Here's how the part is built. I have some questions about the finished solid (model axes, mm). A direction names the side the tool comes from. Round coordinates to 2 decimals unless told otherwise and drop trailing zeros. Write each loop counter-clockwise with the first axis right and the second up, starting at its lowest first coordinate (ties: lowest second). Pieces come first, ordered by that corner, then holes. Notation, with made-up numbers: (9.25, 48) - (31.25, 48) arc R30 cw to (31.25, 71) - close; hole circle Ø8 at (76.25, 38.5). An arc over 180 degrees is marked (long way). Write item = value, one per line. Start each with the question number.
Item 1: If we section it at A-A (z = 9): Please give me the cut outline in (x, y).
Item 2: Which directions (+Z, -Z, +X, -X, +Y, -Y) give clear straight access to the entire face, cutting with the end or side of a thin tool? Please do faces 1 (the face through (5, 13, 1)), 2 (the face through (11.3, 0, 14)), 3 (the face through (-0.635, 22, 14)), 4 (the face through (0, -25, 10)), 5 (the face through (-12.7, -2, 14.4)).
Item 3: If we section it at C-C (x = 1): Please give me the cut outline in (y, z).
Item 4: Thinking about a two-plate mould opening in Y: for faces 6 (the face through (5, 24.5, 16)), 7 (the face through (12.7, -2, 14.4)), 8 (the face through (13.61, 0.03, 12.57)), which applies, pulls with the +Y half, pulls with the -Y half, needs draft (parallel to the pull), parting line crosses it, or undercut?
Item 5: If I drill on line 1 along Y through (x, z) = (10.5, 6.25); line 2 along Y through (x, z) = (2, 15.75); line 3 along Z through (x, y) = (-11, -21.5), over which ranges is the centre line in solid material (lowest first)? Write a range as [from, to].
Item 6: If we section it at B-B (z = 4.75): Please give me the cut outline in (x, y).
Item 7: If we section it at D-D (z = 13.9): Give the number of separate pieces and of enclosed holes in the cut face, and give its area (3 significant figures).
Item 8: For P1, Ø3.5, axis at x = 15, z = 13, coming from the +Y side; P2, Ø1.9, axis at x = 17, z = 15, coming from the -Y side; P3, Ø1.5, axis at x = 30.5, y = 3, coming from the +Z side, each with a flat end and sliding along its axis, tell me the tip position at first contact or that it passes through.
```python
from build123d import *

# Parameters (mm, degrees)
SKETCH_W        = 36
SKETCH_H        = 50
PAD_DEPTH       = 8
PAD001_DEPTH    = 13
SKETCH004_W     = 11
SKETCH004_H     = 4
PAD003_DEPTH    = 13
PAD002_DEPTH    = 13
SKETCH005_W     = 25.977524
SKETCH005_H     = 13
POCKET_DEPTH    = 5
SKETCH006_R     = 1.5
POCKET001_DEPTH = 5
SKETCH007_R     = 1.5
POCKET002_DEPTH = 5
CHAMFER_SIZE    = 2
CHAMFER001_SIZE = 2
CHAMFER002_SIZE = 3
CHAMFER003_SIZE = 2
SKETCH008_W     = 23.210894
SKETCH008_H     = 13
POCKET003_DEPTH = 2
CHAMFER004_SIZE = 1
SKETCH009_W     = 50
SKETCH009_H     = 8
PAD004_DEPTH    = 50
SKETCH010_W     = 50
SKETCH010_H     = 15
POCKET004_DEPTH = 7
SKETCH011_W     = 52.452881
SKETCH011_H     = 55.220252
POCKET005_DEPTH = 8
SKETCH012_W     = 59
SKETCH012_H     = 90
PAD005_DEPTH    = 4
SKETCH013_R     = 19
POCKET006_DEPTH = 4.001
FILLET_R        = 13


with BuildPart() as pad003:
    # Sketch → Pad (new body)
    with BuildSketch(Plane.XY):
        Rectangle(SKETCH_W, SKETCH_H)
    extrude(amount=PAD_DEPTH)

    # Sketch002 → Pad001 (new body)
    with BuildSketch(Plane.XY.offset(8)):
        Polygon((-13.5, -25), (13.5, -25), (13.5, -19.629501), (11.5, -19.629501), (11.5, -23), (-11.5, -23), (-11.5, -18.969727), (-13.5, -18.969727), align=None)
    extrude(amount=PAD001_DEPTH)

    # Sketch004 → Pad003 (new body)
    with BuildSketch(Plane.XY.offset(8)):
        with Locations((4.8652, 22.5)):
            Rectangle(SKETCH004_W, SKETCH004_H)
    extrude(amount=PAD003_DEPTH)


with BuildPart() as fillet_body:
    # Sketch003 → Pad002 (new body)
    with BuildSketch(Plane.XY.offset(8)):
        Polygon((11.3, 2), (18, 2), (18, -5), (16.3, -5), (16.3, -2), (11.3, -2), align=None)
        Polygon((-11.3, 2), (-18, 2), (-18, -5), (-16.3, -5), (-16.3, -2), (-11.3, -2), align=None)
    extrude(amount=PAD002_DEPTH)

    # Fusion: union Pad003
    add(pad003.part)

    # Sketch005 → Pocket (cut)
    with BuildSketch(Plane.XY.offset(8)):
        with Locations((5.011238, 13.5)):
            Rectangle(SKETCH005_W, SKETCH005_H)
    extrude(amount=-POCKET_DEPTH, mode=Mode.SUBTRACT)

    # Sketch006 → Pocket001 (cut)
    with BuildSketch(Plane(origin=(0, 2, 0), x_dir=(-1, 0, 0), z_dir=(0, 1, 0))):
        with Locations((-14.3, 13.9)):
            Circle(SKETCH006_R)
        with Locations((14.3, 13.9)):
            Circle(SKETCH006_R)
    extrude(amount=-POCKET001_DEPTH, mode=Mode.SUBTRACT)

    # Sketch007 → Pocket002 (cut)
    with BuildSketch(Plane(origin=(0, 24.5, 0), x_dir=(-1, 0, 0), z_dir=(0, 1, 0))):
        with Locations((-4.854515, 13.9)):
            Circle(SKETCH007_R)
    extrude(amount=-POCKET002_DEPTH, mode=Mode.SUBTRACT)

    # Chamfer
    chamfer_edges = [fillet_body.edges().sort_by_distance(p)[0] for p in [
        (18, 13.5, 3),
    ]]
    chamfer(chamfer_edges, length=CHAMFER_SIZE)

    # Chamfer001
    chamfer001_edges = [fillet_body.edges().sort_by_distance(p)[0] for p in [
        (16, 13.5, 3),
    ]]
    chamfer(chamfer001_edges, length=CHAMFER001_SIZE)

    # Chamfer002
    chamfer002_edges = [fillet_body.edges().sort_by_distance(p)[0] for p in [
        (14, 13.5, 3),
    ]]
    chamfer(chamfer002_edges, length=CHAMFER002_SIZE)

    # Chamfer003
    chamfer003_edges = [fillet_body.edges().sort_by_distance(p)[0] for p in [
        (11, 13.5, 3),
    ]]
    chamfer(chamfer003_edges, length=CHAMFER003_SIZE)

    # Sketch008 → Pocket003 (cut)
    with BuildSketch(Plane.XY.offset(3)):
        with Locations((7.17125, 13.5)):
            Rectangle(SKETCH008_W, SKETCH008_H)
    extrude(amount=-POCKET003_DEPTH, mode=Mode.SUBTRACT)

    # Chamfer004
    chamfer004_edges = [fillet_body.edges().sort_by_distance(p)[0] for p in [
        (-4.434197, 13.5, 3),
    ]]
    chamfer(chamfer004_edges, length=CHAMFER004_SIZE)

    # Sketch009 → Pad004 (new body)
    with BuildSketch(Plane.YZ.offset(18)):
        with Locations((0, 4)):
            Rectangle(SKETCH009_W, SKETCH009_H)
    extrude(amount=PAD004_DEPTH)

    # Sketch010 → Pocket004 (cut)
    with BuildSketch(Plane.XY.offset(8)):
        with Locations((17, 12.5)):
            Rectangle(SKETCH010_W, SKETCH010_H)
    extrude(amount=-POCKET004_DEPTH, mode=Mode.SUBTRACT)

    # Sketch011 → Pocket005 (cut)
    with BuildSketch(Plane.XY.offset(8)):
        with Locations((45.22644, 0)):
            Rectangle(SKETCH011_W, SKETCH011_H)
    extrude(amount=-POCKET005_DEPTH, mode=Mode.SUBTRACT)

    # Sketch012 → Pad005 (new body)
    with BuildSketch(Plane(origin=(0, 0, 0), x_dir=(1, 0, 0), z_dir=(0, 0, -1))):
        with Locations((11.5, 0)):
            Rectangle(SKETCH012_W, SKETCH012_H)
    extrude(amount=PAD005_DEPTH)

    # Sketch013 → Pocket006 (cut, through all)
    with BuildSketch(Plane.XY):
        with Locations((-18, 45)):
            Circle(SKETCH013_R)
        with Locations((-18, -45)):
            Circle(SKETCH013_R)
    extrude(amount=-POCKET006_DEPTH, mode=Mode.SUBTRACT)

    # Fillet
    fillet_edges = [fillet_body.edges().sort_by_distance(p)[0] for p in [
        (1, -45, -2),
        (1, 45, -2),
    ]]
    fillet(fillet_edges, radius=FILLET_R)


solid = fillet_body.part
```
Reply:
q1.outline = (-18, -5) - (-16.3, -5) - (-16.3, -2) - (-11.3, -2) - (-11.3, 2) - (-18, 2) - close; (-13.5, -25) - (13.5, -25) - (13.5, -19.63) - (11.5, -19.63) - (11.5, -23) - (-11.5, -23) - (-11.5, -18.97) - (-13.5, -18.97) - close; (-0.63, 20.5) - (10.37, 20.5) - (10.37, 24.5) - (-0.63, 24.5) - close; (11.3, -2) - (16.3, -2) - (16.3, -5) - (18, -5) - (18, 2) - (11.3, 2) - close
q2.face_1 = +Z, +X
q2.face_2 = +Z, +Y
q2.face_3 = +Z, -X, +Y
q2.face_4 = +Z, +X, -X, -Y
q2.face_5 = +Z
q3.outline = (-40.01, -4) - (40.01, -4) - (40.01, 0) - (25, 0) - (25, 8) - (24.5, 8) - (24.5, 21) - (20.5, 21) - (20.5, 8) - (20, 8) - (20, 1) - (5, 1) - (5, 8) - (-23, 8) - (-23, 21) - (-25, 21) - (-25, 0) - (-40.01, 0) - close
q4.face_6 = pulls with the +Y half
q4.face_7 = undercut
q4.face_8 = needs draft
q5.line_1 = [-25, 5], [20, 25]
q5.line_2 = [-25, -23], [20.5, 24.5]
q5.line_3 = [-4, 8]
q6.outline = (-18, -25) - (19, -25) - (19, 5) - (-8, 5) - (-8, 20) - (19, 20) - (19, 25) - (-18, 25) - close
q7.separate_pieces = 7
q7.enclosed_holes = 0
q7.area = 141 mm2
q8.P1 = 2
q8.P2 = -5
q8.P3 = 0
